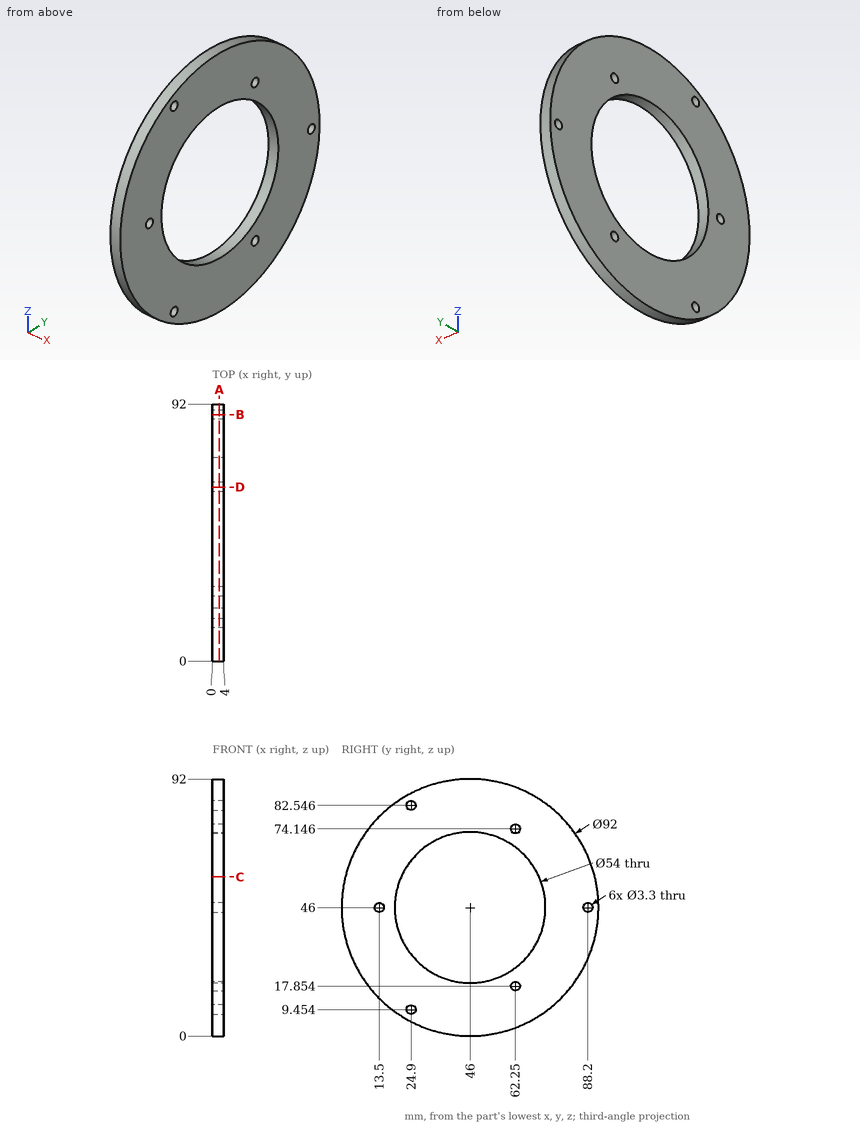
Study the drawing (mm; zero at the part's minimum x, y, z) and answer. Round coordinates to 2 decimals unless told otherwise and drop trailing zeros. Write each loop counter-clockwise with the first axis right and the second up, starting at its lowest first coordinate (ties: lowest second). Pieces come first, ordered by that corner, then holes. Notation, with made-up numbers: (-3.5, 11) -> (25.5, 11) arc R36 ccw to (25.5, 50) -> close; hole circle Ø10 at (13.25, 5.5). An arc over 180 degrees is marked (long way). Answer as CSV lines item,"result". Start each with the question number.
(1) Find the intervals of material crossed by probe 1 along Y at (x, z) = (2.5, 46); probe 2 along Z at (x, y) = (2.2, 62.25) (1 decimal); probe 3 along Z at (x, y) = (2, 47), in increasing order.
(2) The part is cut by section C-C, the plane z = 57. Give the vertices of the cut face in (x, y) (1 decimal).
(3) The part is cut by section D-D, the plane y = 62.25. Give the vertices of the cut face in (x, z).
(4) The part is cut by section B-B, the plane y = 88.2. Give the vertices of the cut face in (x, z), then the cut area to 3 significant figures.
(5) The part is cut by section A-A, the plane x = 2.5. Give the vertices of the cut face in (y, z).
(6) Each of these flat-tipped pins is pushed along its axis until it touches: pin 1 (2 mm diameter, centred on y = 62.25, z = 74.15, fed in from -X); pin 2 (2 mm diameter, centred on x = 1, z = 43, fed in from +Y). Where does it stop, or does it pass through?
Output values:
1,probe 1,"y = 0 to 11.85, 15.15 to 19, 73 to 86.55, 89.85 to 92"
1,probe 2,"z = 3 to 16.2, 19.5 to 24.4, 67.6 to 72.5, 75.8 to 89"
1,probe 3,"z = 0.01 to 19.02, 72.98 to 91.99"
2,outline,"(0, 1.3) -> (4, 1.3) -> (4, 21.3) -> (0, 21.3) -> close; (0, 70.7) -> (4, 70.7) -> (4, 90.7) -> (0, 90.7) -> close"
3,outline,"(0, 2.97) -> (4, 2.97) -> (4, 16.2) -> (0, 16.2) -> close; (0, 19.5) -> (4, 19.5) -> (4, 24.44) -> (0, 24.44) -> close; (0, 67.56) -> (4, 67.56) -> (4, 72.5) -> (0, 72.5) -> close; (0, 75.8) -> (4, 75.8) -> (4, 89.03) -> (0, 89.03) -> close"
4,outline,"(0, 27.69) -> (4, 27.69) -> (4, 44.35) -> (0, 44.35) -> close; (0, 47.65) -> (4, 47.65) -> (4, 64.31) -> (0, 64.31) -> close"
4,area,"133 mm²"
5,outline,"circle Ø92 at (46, 46); hole circle Ø3.3 at (13.5, 46); hole circle Ø54 at (46, 46); hole circle Ø3.3 at (24.9, 9.45); hole circle Ø3.3 at (24.9, 82.55); hole circle Ø3.3 at (62.25, 17.85); hole circle Ø3.3 at (62.25, 74.15); hole circle Ø3.3 at (88.2, 46)"
6,pin 1,"passes through"
6,pin 2,"stops at y = 91.96"
